```python
from build123d import *

# Parameters (mm, degrees)
SKETCH_1_W          = 30
SKETCH_1_H          = 22
EXTRUDE_1_DEPTH     = 4
SKETCH_2_W          = 30
SKETCH_2_H          = 4
EXTRUDE_2_DEPTH     = 18
SKETCH_3_R          = 2
CUT_EXTRUDE_1_DEPTH = 20
SKETCH_4_R          = 2
CUT_EXTRUDE_2_DEPTH = 20
CHAMFER_1_SIZE      = 6
FILLET_1_R          = 8


with BuildPart() as part:
    # 草图1 → 凸台-拉伸1 (new body)
    with BuildSketch(Plane(origin=(0, 0, 0), x_dir=(1, 0, 0), z_dir=(0, 1, 0))):
        with Locations((15, -11)):
            Rectangle(SKETCH_1_W, SKETCH_1_H)
    extrude(amount=EXTRUDE_1_DEPTH)

    # 草图2 → 凸台-拉伸2 (add)
    with BuildSketch(Plane(origin=(0, 4, 0), x_dir=(1, 0, 0), z_dir=(0, 1, 0))):
        with Locations((15, -2)):
            Rectangle(SKETCH_2_W, SKETCH_2_H)
    extrude(amount=EXTRUDE_2_DEPTH)

    # 草图3 → 切除-拉伸1 (cut)
    with BuildSketch(Plane(origin=(0, 4, 0), x_dir=(1, 0, 0), z_dir=(0, 1, 0))):
        with Locations(Location((8, -14, 0), (0, 0, 270))):
            Circle(SKETCH_3_R)
        with Locations(Location((22, -14, 0), (0, 0, 270))):
            Circle(SKETCH_3_R)
    extrude(amount=-CUT_EXTRUDE_1_DEPTH, mode=Mode.SUBTRACT)

    # 草图4 → 切除-拉伸2 (cut)
    with BuildSketch(Plane.XY.offset(4)):
        with Locations((8, 14)):
            Circle(SKETCH_4_R)
        with Locations((22, 14)):
            Circle(SKETCH_4_R)
    extrude(amount=-CUT_EXTRUDE_2_DEPTH, mode=Mode.SUBTRACT)

    # 倒角1
    chamfer_1_edges = [part.edges().sort_by_distance(p)[0] for p in [
        (15, 4, 4),
    ]]
    chamfer(chamfer_1_edges, length=CHAMFER_1_SIZE)

    # 圆角1
    fillet_1_edges = [part.edges().sort_by_distance(p)[0] for p in [
        (0, 22, 2),
        (30, 22, 2),
        (30, 2, 22),
        (0, 2, 22),
    ]]
    fillet(fillet_1_edges, radius=FILLET_1_R)


solid = part.part
```
Could you check a few things on this model? Use its own coordinates, in mm. A direction names the side the tool comes from. Round coordinates to 2 decimals unless told otherwise and drop trailing zeros. Loops run counter-clockwise (first coordinate to the right, second up) from the corner with the lowest first, then second, coordinate; pieces in that order, holes last. Notation, with made-up numbers: (38, -7.75) -> (76, -7.75) arc R19 ccw to (76, 2.25) -> close; hole circle Ø10 at (-23, -39.75). An arc over 180 degrees is marked (long way). Put each result on its own line as item: value.
Q1. I want a section at B-B on y = 14.75. Write out the boundary of the cut face in (x, z).
Checks:
outline: (0.04, 0) -> (6.15, 0) -> (6.15, 4) -> (0.04, 4) -> close; (9.85, 0) -> (20.15, 0) -> (20.15, 4) -> (9.85, 4) -> close; (23.85, 0) -> (29.96, 0) -> (29.96, 4) -> (23.85, 4) -> close
Q2. I want a section at D-D on x = 6.5. Write out the boundary of the cut face in (y, z), and give its area (3 significant figures).
Checks:
outline: (0, 0) -> (12.68, 0) -> (12.68, 4) -> (10, 4) -> (4, 10) -> (4, 12.68) -> (0, 12.68) -> close; (0, 15.32) -> (4, 15.32) -> (4, 21.86) -> (0, 21.86) -> close; (15.32, 0) -> (21.86, 0) -> (21.86, 4) -> (15.32, 4) -> close
area: 156 mm2
Q3. Please list where these lines run through material, in increasing order: line 1 (Y direction, x = 22, z = 2.95); line 2 (X direction, y = 12.5, z = 2.75); line 3 (Y direction, x = 21, z = 18.5). Write a range as from..to.
Checks:
line 1: 0..12, 16..22
line 2: 0..6.68, 9.32..20.68, 23.32..30
line 3: 0..4
Q4. I want a section at A-A on x = 18. Write out the boundary of the cut face in (y, z), and give its area (3 significant figures).
Checks:
outline: (0, 0) -> (22, 0) -> (22, 4) -> (10, 4) -> (4, 10) -> (4, 22) -> (0, 22) -> close
area: 178 mm2
Q5. For pin 1 Ø6.5 at (x, y) = (8, 14) entering from +Z; pin 2 Ø3 at (x, z) = (22, 14) entering from +Y; pin 3 Ø12 at (x, y) = (4.5, 13) entering from +Z; pin 4 Ø2 at (x, z) = (22.5, 17) entering from +Y, each with a flat end and sliding along its axis, tell me the tip position at first contact or that it passes through.
Checks:
pin 1: z = 4
pin 2: through
pin 3: z = 7
pin 4: y = 4
Q6. Which directions (+Z, -Z, +X, -X, +Y, -Y) give clear straight access to the entire face, cutting with the end or side of a thin tool? Please do faces 1 (the flat face through (0, 5, 6)), 2 (the flat face through (15, 4, 16)).
Checks:
face 1: +Z, -Z, -X, +Y, -Y
face 2: +Z, +X, -X, +Y
Q7. Thinking about a two-plate mould opening in X: for faces 3 (the cylindrical face through (20.8, 2, 12.4)), 4 (the flat face through (15, 0, 11)), 5 (the cylindrical face through (2.281, 19.594, 1.972)), which applies, pulls with the +X half, pulls with the -X half, needs draft (parallel to the pull), parting line crosses it, or undercut?
Checks:
face 3: undercut
face 4: needs draft
face 5: pulls with the -X half
Q8. I want a section at C-C on y = 1.75. Write out the boundary of the cut face in (x, z), and give its area (3 significant figures).
Checks:
outline: (0, 0) -> (30, 0) -> (30, 14) arc R8 ccw to (22, 22) -> (8, 22) arc R8 ccw to (0, 14) -> close; hole circle Ø4 at (8, 14); hole circle Ø4 at (22, 14)
area: 607 mm2
